```python
from build123d import *

# Parameters (mm, degrees)
F1_DEPTH = 30
F2_T     = -3


with BuildPart() as f1:
    # F0 (on Top) → F1 (new body)
    with BuildSketch(Plane.XY):
        Polygon((-20, 70), (-65, 70), (-65, 45), (-60, 45), (-60, -35), (-36.6666666667, -70), (0, -70), (36.6666666667, -70), (60, -35), (60, 45), (65, 45), (65, 70), (20, 70), (20, 45), (25, 45), (25, -24.4028526794), (17.9352351196, -35), (0, -35), (-17.9352351196, -35), (-25, -24.4028526794), (-25, 45), (-20, 45), align=None)
    extrude(amount=F1_DEPTH)

    # F2
    f2_openings = [f1.faces().sort_by_distance(p)[0] for p in [
        (23.057247, -30.76118, 30),
    ]]
    offset(amount=F2_T, openings=f2_openings, kind=Kind.INTERSECTION)


solid = f1.part
```
The listing builds one solid part. Answer for the finished solid, in the listing's coordinates (mm). A direction names the side the tool comes from. Give positions to 0.01 mm unless a question says otherwise; leave off trailing zeros. Order: outer loops, then holes, each group sorted by start corner. A loop starts at its lowest first (then second) coordinate and runs counter-clockwise, first axis right, second up. Notation, with made-up numbers: (10.5, 42.5) -> (69.5, 42.5) arc R29 ccw to (69.5, 75.5) -> close; hole circle Ø6 at (-35, 21.25). An arc over 180 degrees is marked (long way). One line per item, written item: value.
1) Find section D-D, the plane y = -57. Determine the outline of the cut face in (x, z), plus the area to 3 significant figures.
Reported:
outline: (-45.33, 0) -> (45.33, 0) -> (45.33, 30) -> (41.73, 30) -> (41.73, 3) -> (-41.73, 3) -> (-41.73, 30) -> (-45.33, 30) -> close
area: 467 mm^2
2) A tool of negligible diameter and unlimited length cuts with its end or side. For faces 4 (the flat face through (21.517, -29.627, 14.79)), 5 (the flat face through (-23.711, -31.744, 16.311)), from which of +Z, -Z, +X, -X, +Y, -Y can it reach the whole face along a straight path? Write none if from no direction.
Reported:
face 4: +Z, -Z
face 5: +Z
3) Find section B-B, the plane x = 4.5. Determine the outline of the cut face in (y, z), plus the area to 3 significant figures.
Reported:
outline: (-70, 0) -> (-35, 0) -> (-35, 30) -> (-38, 30) -> (-38, 3) -> (-67, 3) -> (-67, 30) -> (-70, 30) -> close
area: 267 mm^2
4) Find the intervals of material crossed by line 1 (X direction, y = 22, z = 11.5); line 2 (X direction, y = 58, z = 5); line 3 (Y direction, x = 20.5, z = 23.5), in increasing order.
Reported:
line 1: x = -60 to -57, -28 to -25, 25 to 28, 57 to 60
line 2: x = -65 to -62, -23 to -20, 20 to 23, 62 to 65
line 3: y = -70 to -67, -36.56 to -31.15, 45 to 70
5) Flat-ended cylindrical pins translate along their axes: P1, Ø2, axis at x = -41, z = 15, coming from the -Y side; P2, Ø15, axis at y = 22.5, z = 21, coming from the -X side; P3, Ø10, axis at y = -41.5, z = 5.5, coming from the +X side. Find the tip coordinate at first contact, or state that the pin passes through.
Reported:
P1: stops at y = -65
P2: stops at x = -60
P3: stops at x = 59
6) Find section C-C, the plane y = 59.5. Determine the outline of the cut face in (x, z).
Reported:
outline: (-65, 0) -> (-20, 0) -> (-20, 30) -> (-23, 30) -> (-23, 3) -> (-62, 3) -> (-62, 30) -> (-65, 30) -> close; (20, 0) -> (65, 0) -> (65, 30) -> (62, 30) -> (62, 3) -> (23, 3) -> (23, 30) -> (20, 30) -> close
7) Determine the mould class of faces 1 (the flat face through (-24.4, -25.6, 30)), 2 (the flat face through (-42, 70, 15)), 3 (the flat face through (57, 6, 16)) for opening direction Y: pulls with the +Y half, pulls with the -Y half, needs draft (parallel to the pull), parting line crosses it, or undercut.
Reported:
face 1: needs draft
face 2: pulls with the +Y half
face 3: undercut
8) Find section A-A, the plane y = 23.5. Determine the outline of the cut face in (x, z), plus the area to 3 significant figures.
Reported:
outline: (-60, 0) -> (-25, 0) -> (-25, 30) -> (-28, 30) -> (-28, 3) -> (-57, 3) -> (-57, 30) -> (-60, 30) -> close; (25, 0) -> (60, 0) -> (60, 30) -> (57, 30) -> (57, 3) -> (28, 3) -> (28, 30) -> (25, 30) -> close
area: 534 mm^2
